Autodesk Inventor part; units mm, degrees
ref_plane "YZ Plane" through (0, 0, 0) normal (1, 0, 0) x (0, 1, 0)
ref_plane "XZ Plane" through (0, 0, 0) normal (0, 1, 0) x (-1, 0, 0)
ref_plane "XY Plane" through (0, 0, 0) normal (0, 0, 1) x (1, 0, 0)
sketch "Sketch1" plane through (0, 0, 0) normal (0, 1, 0) x (-1, 0, 0)
  arc A0 (11.5434, 7) -> (11.5434, -7) centre (0, 0) ccw
  line L0 (13.5, -7) -> (13.5, 7)
  line L1 (13.5, -7) -> (11.5434, -7)
  line L2 (13.5, 7) -> (11.5434, 7)
  dimension "d0" = 27
  dimension "d2" = 14
extrude "Extrusion1" add sketch "Sketch1" along normal blind 15
sketch "Sketch2" plane through (0, 15, 0) normal (0, 1, 0) x (1, 0, 0)
  arc A0 (-11.5434, -7) -> (-11.5434, 7) centre (0, 0) ccw
  circle A1 centre (0, 0) radius 11
  dimension "d6" = 22
extrude "Extrusion2" add sketch "Sketch2" along normal blind 2
sketch "Sketch3" plane through (0, 17, 0) normal (0, 1, 0) x (1, 0, 0)
  circle A0 centre (0, 0) radius 9.5
  dimension "d9" = 19
extrude "Extrusion3" add sketch "Sketch3" along normal blind 2
fillet "Fillet1" radius 1 1 edges at (-9.5, 17, 0)
sketch "Sketch4" plane through (0, 19, 0) normal (0, 1, 0) x (1, 0, 0)
  circle A0 centre (0, 0) radius 9.5
  circle A1 centre (0, 0) radius 10
  dimension "d13" = 20
extrude "Extrusion4" add sketch "Sketch4" along normal blind 16 contours A0
sketch "Sketch5" plane through (0, 35, 0) normal (0, 1, 0) x (1, 0, 0)
  circle A0 centre (0, 0) radius 9.5
  line L0 (0, 0) -> (8, 0) construction
  line L1 (0, -8) -> (-19.2017, -8)
  line L2 (-19.2017, -8) -> (-19.2017, -21.9067)
  line L3 (-19.2017, -21.9067) -> (19.6427, -21.9067)
  line L4 (19.6427, -21.9067) -> (19.6427, -8)
  line L5 (19.6427, -8) -> (0, -8)
  line L6 (0, 8) -> (-19.2017, 8)
  line L7 (-19.2017, 8) -> (-19.2017, 24.6239)
  line L8 (-19.2017, 24.6239) -> (24.0089, 24.6239)
  line L9 (0, 8) -> (27.6995, 8)
  line L10 (27.6995, 8) -> (27.6995, 24.6239)
  line L11 (27.6995, 24.6239) -> (24.0089, 24.6239)
extrude "Extrusion5" cut sketch "Sketch5" against normal blind 29 contours L9 L6 A0 | A0 L6 L7 L8 L11 L10 L9 | L5 L4 L3 L2 L1 A0 | A0 L1 L5
sketch "Sketch6" plane through (-13.5, 0, -7) normal (-1, 0, 0) x (0, 0, 1)
  circle A0 centre (7, 7.5) radius 4.5
  point P0 (7, 0)
  dimension "d21" = 9
extrude "Extrusion6" cut sketch "Sketch6" against normal blind 19
sketch "Sketch7" plane through (0, 0, 0) normal (0, -1, 0) x (1, 0, 0)
  circle A0 centre (0, 0) radius 7.5
  dimension "d26" = 15
extrude "Extrusion7" cut sketch "Sketch7" against normal blind 12
thread "Thread1"
thread "Thread2"
fillet "Fillet2" radius 0.3 4 edges at (9.5, 35, 0) (-9.5, 35, 0) (0, 35, 8) (0, 35, -8)
thread "Thread3"
sketch "Sketch8" plane through (-10.8743, 6, 8) normal (0, 0, 1) x (1, 0, 0)
  circle A0 centre (10.8743, 11) radius 5
  point P0 (10.8743, -6)
  dimension "d34" = 10
extrude "Extrusion8" cut sketch "Sketch8" against normal blind 20
sketch "Sketch9" plane through (0, 0, 0) normal (0, -1, 0) x (1, 0, 0)
  point P0 (0, 0)
properties part number "zadnji deo klipa" material "ABS Plastic"
Geometry check sheet. Reference: the model listing, model coordinates, mm. A direction names the side the tool comes from. Give positions to 0.01 mm unless a question says otherwise; leave off trailing zeros. Order: outer loops, then holes, each group sorted by start corner. A loop starts at its lowest first (then second) coordinate and runs counter-clockwise, first axis right, second up. Notation, with made-up numbers: (-4.75, 4.25) - (15.25, 4.25) arc R34 ccw to (15.25, 37.25) - close; hole circle Ø6 at (-14.5, 7.5). An arc over 180 degrees is marked (long way). Answer as a JSON object with one key per item and string values.
(1) Cross-section at B-B (x = -4.25). Record the cut outline in (y, z).
Report:
{"outline": "(0, -12.81) - (6, -12.81) - (6, -8) - (14.37, -8) - (14.37, 8) - (6, 8) - (6, 12.81) - (0, 12.81) - (0, 6.18) - (12, 6.18) - (12, -6.18) - (0, -6.18) - close; (19.63, -8) - (34.7, -8) arc R0.3 ccw to (35, -7.7) - (35, 7.7) arc R0.3 ccw to (34.7, 8) - (19.63, 8) - close"}
(2) Cross-section at D-D (z = -1.75). State how many separate pieces and enclosed holes the cut face has, then the cut area to 3 significant figures.
Report:
{"separate pieces": "2", "enclosed holes": "1", "area": "478 mm^2"}
(3) Depth check by flat-ended pin: pin 1 Ø1.7 at (x, z) = (0.5, -11) entering from +Y; pin 2 Ø4 at (y, z) = (30, -1.5) entering from -X; pin 3 Ø4.5 at (x, z) = (1.5, -3.5) entering from -Y. Enter the tip coordinate at first touch or a pass-through.
Report:
{"pin 1": "y = 6", "pin 2": "x = -9.5", "pin 3": "y = 12"}
(4) Cross-section at C-C (y = 7.5). Record the cut outline in (x, z), then the cut area to 3 significant figures.
Report:
{"outline": "(-13.5, -7) - (-11.54, -7) arc R13.5 ccw to (-10.87, -8) - (10.87, -8) arc R13.5 ccw to (10.87, 8) - (-10.87, 8) arc R13.5 ccw to (-11.54, 7) - (-13.5, 7) - (-13.5, 4.5) - (-6, 4.5) arc R7.5 cw (long way) to (-6, -4.5) - (-13.5, -4.5) - close", "area": "179 mm^2"}
(5) Tool access check on faces 5 (the flat face through (10.8, 17, 0)), 6 (the cylindrical face through (-9.5, 26.2, 0.1)), 7 (the cylindrical face through (-9.8, 5.78, 4.16)), 8 (the flat face through (2, 12, 0)), 9 (the flat face through (0, 24, -8)). Record the directions out of +Z, -Z, +X, -X, +Y, -Y that give a thin tool (end or side, any length) a straight path to the whole face; none if there is none.
Report:
{"face 5": "+X, +Y", "face 6": "-X, +Y", "face 7": "-X", "face 8": "-Y", "face 9": "-Z, +X, -X, +Y"}
(6) Material ranges on line 1 (Z direction, x = -9.5, y = 7.5); line 2 (X direction, y = 6.5, z = 0); line 3 (Y direction, x = -8, z = 0), recorded low to high.
Report:
{"line 1": "-8 to -4.5, 4.5 to 8", "line 2": "7.5 to 13.5", "line 3": "0 to 3, 12 to 35"}
(7) Cross-section at A-A (y = 21). Record the cut outline in (x, z), then the cut area to 3 significant figures.
Report:
{"outline": "(-5.12, -8) - (-3, -8) - (-3, 8) - (-5.12, 8) arc R9.5 ccw to start; (3, -8) - (5.12, -8) arc R9.5 ccw to (5.12, 8) - (3, 8) - close", "area": "167 mm^2"}
(8) Draft check along X on faces 1 (the cylindrical face through (9.5, 26.2, -0.1)), 2 (the cylindrical face through (6.93, 5.92, -2.87)), 3 (the cylindrical face through (2.307, 12.564, 0.112)), 4 (the flat face through (0, 24, 8)). Enter one of: released by +X, released by -X, zero draft, split by the parting line, or undercut.
Report:
{"face 1": "released by +X", "face 2": "undercut", "face 3": "undercut", "face 4": "zero draft"}
